Model file for the job. Use its own axes, mm. Face numbers are marked on the shaded views. A direction names the side the tool comes from. Give positions to 0.01 mm unless a question says otherwise; leave off trailing zeros. Write each loop counter-clockwise with the first axis right and the second up, starting at its lowest first coordinate (ties: lowest second). Pieces come first, ordered by that corner, then holes. Notation, with made-up numbers: (53, 74.25) - (93, 74.25) arc R27 ccw to (93, 106.25) - close; hole circle Ø10 at (-0.5, 82.5). An arc over 180 degrees is marked (long way). Use CSV: the item, a comma, the result in double quotes.
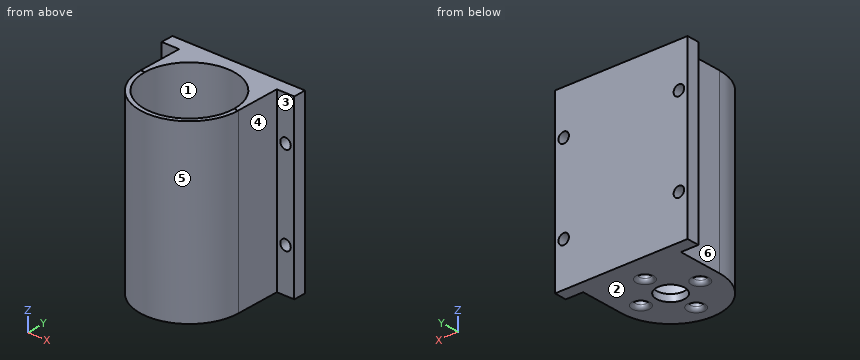
from build123d import *

# Parameters (mm, degrees)
SKETCH1_R           = 14
BOSS_EXTRUDE1_DEPTH = 50
SKETCH5_W           = 28
SKETCH5_H           = 50.034880911
BOSS_EXTRUDE2_DEPTH = 21
SKETCH2_R           = 12.791811967
CUT_EXTRUDE1_DEPTH  = 48
SKETCH3_R           = 4
CUT_EXTRUDE2_DEPTH  = 49
SKETCH4_R           = 1.5
CUT_EXTRUDE3_DEPTH  = 49
SKETCH6_R           = 12.79
CUT_EXTRUDE5_DEPTH  = 21
SKETCH7_W           = 28
SKETCH7_H           = 4.634699127
CUT_EXTRUDE6_DEPTH  = 53
SKETCH8_W           = 50.034880911
SKETCH8_H           = 3.58
BOSS_EXTRUDE3_DEPTH = 5
SKETCH13_R          = 1.5
CUT_EXTRUDE7_DEPTH  = 5
SKETCH14_W          = 50.034880911
SKETCH14_H          = 3.58
BOSS_EXTRUDE4_DEPTH = 5
SKETCH15_R          = 1.5
CUT_EXTRUDE8_DEPTH  = 5
FILLET1_R           = 1
FILLET2_R           = 1


with BuildPart() as part:
    # Sketch1 → Boss-Extrude1 (new body)
    with BuildSketch(Plane.XY):
        Circle(SKETCH1_R)
    extrude(amount=BOSS_EXTRUDE1_DEPTH)

    # Sketch5 → Boss-Extrude2 (add)
    with BuildSketch(Plane(origin=(0, 0, 0), x_dir=(1, 0, 0), z_dir=(0, 1, 0))):
        with Locations((0, -25.017440456)):
            Rectangle(SKETCH5_W, SKETCH5_H)
    extrude(amount=BOSS_EXTRUDE2_DEPTH)

    # Sketch2 → Cut-Extrude1 (cut)
    with BuildSketch(Plane.XY.offset(50)):
        Circle(SKETCH2_R)
    extrude(amount=-CUT_EXTRUDE1_DEPTH, mode=Mode.SUBTRACT)

    # Sketch3 → Cut-Extrude2 (cut)
    with BuildSketch(Plane(origin=(0, 0, 0), x_dir=(-1, 0, 0), z_dir=(0, 0, -1))):
        Circle(SKETCH3_R)
    extrude(amount=-CUT_EXTRUDE2_DEPTH, mode=Mode.SUBTRACT)

    # Sketch4 → Cut-Extrude3 (cut)
    with BuildSketch(Plane(origin=(0, 0, 0), x_dir=(-1, 0, 0), z_dir=(0, 0, -1))):
        with Locations((0, -8.5)):
            Circle(SKETCH4_R)
        with Locations((0, 8.5)):
            Circle(SKETCH4_R)
        with Locations((8.5, 0)):
            Circle(SKETCH4_R)
        with Locations((-8.5, 0)):
            Circle(SKETCH4_R)
    extrude(amount=-CUT_EXTRUDE3_DEPTH, mode=Mode.SUBTRACT)

    # Sketch6 → Cut-Extrude5 (cut)
    with BuildSketch(Plane.XY.offset(50.034880911)):
        Circle(SKETCH6_R)
    extrude(amount=-CUT_EXTRUDE5_DEPTH, mode=Mode.SUBTRACT)

    # Sketch7 → Cut-Extrude6 (cut)
    with BuildSketch(Plane.XY.offset(50.034880911)):
        with Locations((0, 18.682650437)):
            Rectangle(SKETCH7_W, SKETCH7_H)
    extrude(amount=-CUT_EXTRUDE6_DEPTH, mode=Mode.SUBTRACT)

    # Sketch8 → Boss-Extrude3 (add)
    with BuildSketch(Plane(origin=(14, 0, 0), x_dir=(0, 0, -1), z_dir=(1, 0, 0))):
        with Locations((-25.017440456, 14.575300873)):
            Rectangle(SKETCH8_W, SKETCH8_H)
    extrude(amount=BOSS_EXTRUDE3_DEPTH)

    # Sketch13 → Cut-Extrude7 (cut)
    with BuildSketch(Plane.XZ.offset(-12.785300873)):
        with Locations((16.5, 37.526160683)):
            Circle(SKETCH13_R)
        with Locations((16.5, 12.508720228)):
            Circle(SKETCH13_R)
    extrude(amount=-CUT_EXTRUDE7_DEPTH, mode=Mode.SUBTRACT)

    # Sketch14 → Boss-Extrude4 (add)
    with BuildSketch(Plane.ZY.offset(14)):
        with Locations((25.017440456, 14.575300873)):
            Rectangle(SKETCH14_W, SKETCH14_H)
    extrude(amount=BOSS_EXTRUDE4_DEPTH)

    # Sketch15 → Cut-Extrude8 (cut)
    with BuildSketch(Plane.XZ.offset(-12.785300873)):
        with Locations((-16.5, 12.508720228)):
            Circle(SKETCH15_R)
        with Locations((-16.5, 37.526160683)):
            Circle(SKETCH15_R)
    extrude(amount=-CUT_EXTRUDE8_DEPTH, mode=Mode.SUBTRACT)

    # Fillet1
    fillet1_edges = [part.edges().sort_by_distance(p)[0] for p in [
        (10, 0, 0),
    ]]
    fillet(fillet1_edges, radius=FILLET1_R)

    # Fillet2
    fillet2_edges = [part.edges().sort_by_distance(p)[0] for p in [
        (1.5, -8.5, 0),
        (1.5, 8.5, 0),
        (-7, 0, 0),
    ]]
    fillet(fillet2_edges, radius=FILLET2_R)


solid = part.part
(1) Wall check: probe 1 along Y at (x, z) = (0, 1.75); probe 2 along Z at (x, y) = (-16, 13); probe 3 along X at (y, z) = (0, 33.5). Give the ranges that are in metal, low to high. Write a range as [from, to].
Checked values:
probe 1,"y = [-14, -10], [-7, -4], [4, 7], [10, 16.37]"
probe 2,"z = [0, 11.09], [13.92, 36.11], [38.94, 50.03]"
probe 3,"x = [-14, -12.79], [12.79, 14]"
(2) Pull direction Y, two halves, no side cores. Call the marked faces 1, 2 and 3: released by +Y, released by -Y, zero draft, split by the parting line, or undercut.
Checked values:
face 1,"undercut"
face 2,"zero draft"
face 3,"released by -Y"
(3) Flat gauge pins, fed straight in: P1, Ø1, axis at y = 3, z = 16.5, coming from the -X side; P2, Ø1.5, axis at x = 12, z = 38, coming from the -Y side; P3, Ø13, axis at x = 0, y = 0, coming from the +Z side. Where does each tip first touch, or does it go through?
Checked values:
P1,"stops at x = -14"
P2,"stops at y = -8.33"
P3,"stops at z = 2"
(4) 3-axis set-ups, long thin cutter, end or side, ignore diameter. For the marked faces 4, 5 and 6: which of +Z, -Z, +X, -X, +Y, -Y reach the whole face in a straight line?
Checked values:
face 4,"+Z, -Z, +X, -Y"
face 5,"+Z, -Z, -Y"
face 6,"+Z, -Z, -X, -Y"
(5) Saw through at C-C, the plane y = -8.5. List the corners of the cut face in (x, z), then the cut area to 3 significant figures.
Checked values:
outline,"(-11.12, 0) - (-2.5, 0) arc R1 ccw to (-1.5, 1) - (-1.5, 2) - (-9.56, 2) - (-9.56, 50) - (-11.12, 50) - close; (1.5, 1) arc R1 ccw to (2.5, 0) - (11.12, 0) - (11.12, 50) - (9.56, 50) - (9.56, 2) - (1.5, 2) - close"
area,"188 mm^2"
(6) Saw through at A-A, the plane x = -16.5. List the corners of the cut face in (y, z), then the cut area to 3 significant figures.
Checked values:
outline,"(12.79, 0) - (16.37, 0) - (16.37, 11.01) - (12.79, 11.01) - close; (12.79, 14.01) - (16.37, 14.01) - (16.37, 36.03) - (12.79, 36.03) - close; (12.79, 39.03) - (16.37, 39.03) - (16.37, 50.03) - (12.79, 50.03) - close"
area,"158 mm^2"
(7) Saw through at B-B, the plane z = 40. List the corners of the cut face in (x, y).
Checked values:
outline,"(-19, 12.79) - (-14, 12.79) - (-14, 0) arc R14 ccw to (14, 0) - (14, 12.79) - (19, 12.79) - (19, 16.37) - (-19, 16.37) - close; hole circle Ø25.58 at (0, 0)"
